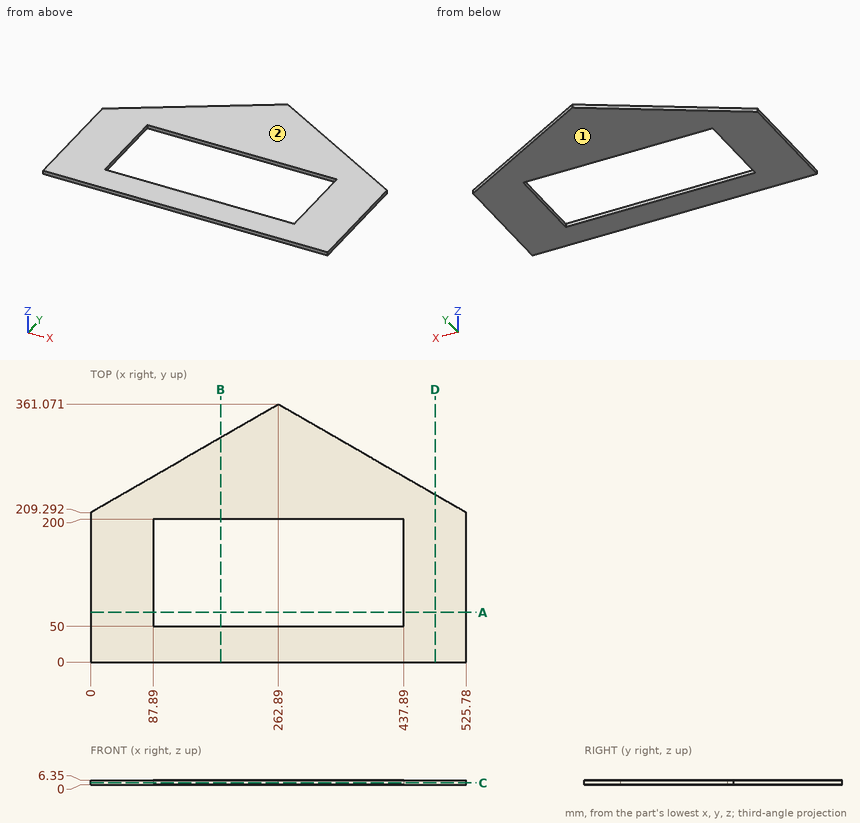
Print and shaded views of the part. All mm, measured from the part's lowest x, y and z. Coordinates: 2 decimals unless noted, no trailing zeros. Order: outer loops, then holes, each group sorted by start corner. A loop starts at its lowest first (then second) coordinate and runs counter-clockwise, first axis right, second up. Notation, with made-up numbers: M -14,-2.75 L 40,-2.75 A20 ccw 40,7.25 Z; hole C 30,-27.5 d10. An arc over 180 degrees is marked long. One line per question, with ' | ' between items. Start each with the question number.
Q1. Saw through at D-D (x = 482). List the corners of the cut face in (y, z).
Q2. Saw through at C-C (z = 2.5). List the corners of the cut face in (x, y).
Q3. Probe L1, parallel to X at y = 63, z = 3; L2, parallel to Y at x = 263, z = 4; L3, parallel to Y at x = 144.5, z = 3. List the from-to ranges inside material, lowest first. Write a range as from..to.
Q4. Saw through at A-A (y = 69.5). List the corners of the cut face in (x, z), then the cut area to 3 significant figures.
Q5. Two-plate mould, pull along Z, no slides. Class the marked faces 1 and 2: +Z half, -Z half, draft (parallel to the pull), parting line (faces both ways), or undercut.
Q6. Saw through at B-B (x = 182). List the corners of the cut face in (y, z).
Q7. Flat gauge pins, fed straight in: pin 1 Ø1.5 at (x, z) = (161.5, 1.5) entering from +Y; pin 2 Ø1.9 at (x, z) = (302, 4) entering from +Y. Where does each tip first touch, or does it go through?
Check values:
1) outline: M 0,0 L 234.57,0 L 234.57,6.35 L 0,6.35 Z
2) outline: M 0,0 L 525.78,0 L 525.78,209.29 L 262.89,361.07 L 0,209.29 Z; hole M 87.89,50 L 437.89,50 L 437.89,200 L 87.89,200 Z
3) L1: x = 0..87.89, 437.89..525.78 | L2: y = 0..50, 200..361.01 | L3: y = 0..50, 200..292.72
4) outline: M 0,0 L 87.89,0 L 87.89,6.35 L 0,6.35 Z; M 437.89,0 L 525.78,0 L 525.78,6.35 L 437.89,6.35 Z | area: 1,120 mm2
5) face 1: -Z half | face 2: +Z half
6) outline: M 0,0 L 50,0 L 50,6.35 L 0,6.35 Z; M 200,0 L 314.37,0 L 314.37,6.35 L 200,6.35 Z
7) pin 1: stops at y = 302.97 | pin 2: stops at y = 339.04
